Work out the finished part from the listing and answer in its coordinate system (mm). A direction names the side the tool comes from. Round coordinates to 2 decimals unless told otherwise and drop trailing zeros. Write each loop counter-clockwise with the first axis right and the second up, starting at its lowest first coordinate (ties: lowest second). Pieces come first, ordered by that corner, then holes.
1. Determine the mould class of faces 1 (the face through (9, -25, 0)), 2 (the face through (-4, -19, 2.85)), 3 (the face through (-2, -12, 3.5)) for opening direction Y: pulls with the +Y half, pulls with the -Y half, needs draft (parallel to the pull), parting line crosses it, or undercut.
2. Find section D-D (z = 0.5). Count the separate pieces of the cut face and the enclosed holes in it, and give its area (3 significant figures).
3. Straight lines are drawn through the part: probe 1 along Z at (x, y) = (-8.1, -19); probe 2 along Y at (x, z) = (-3, 3); probe 3 along Y at (x, z) = (-3.75, -1). For each, find the intervals that lie inside material, in ascending order.
4. Find section A-A (x = 0). Write down the section's boundary in (y, z), and give its area (3 significant figures).
5. Find section C-C (y = 0). Write down the section's boundary in (x, z), and give its area (3 significant figures).
6. A tool of negligible diameter and unlimited length cuts with its end or side. For faces 4 (the face through (2.53, -19.06, 0.33)), 5 (the face through (-1.49, -8.77, 0.94)), 6 (the face through (3.61, -25.02, -2.05)), 7 (the face through (7, -19, 0)), from which of +Z, -Z, +X, -X, +Y, -Y can it reach the whole face along a straight path? Write none if from no direction.
7. Find section B-B (y = -10). Write down the section's boundary in (x, z).
8. Flat-ended cylindrical pins translate along their axes: pin 1 Ø2 at (x, y) = (-5.5, 1) entering from +Z; pin 2 Ø6.5 at (y, z) = (-9, 0.5) entering from +X; pin 3 Ø2 at (y, z) = (-8.5, 1.5) entering from +X; pin 4 Ø10 at (x, y) = (0, 0) entering from +Z. Find the tip coordinate at first contact, or state that the pin passes through.
```python
from build123d import *

# Parameters (mm, degrees)
SKETCH1_R                      = 6.1
THICKNESS_DEPTH                = 3.5
BOTNUTCUT_START                = -2
SKETCH2_R                      = 2.85
BOTNUTCUT_DEPTH                = 2.6
SKETCH3_R                      = 1.55
BOTSCREWCUT_DEPTH              = 2
CUT_EXTRUDE1_START             = -7
CUT_EXTRUDE1_DEPTH             = 7
RAILNUTCUT_START               = -2
RAILNUTCUT_DEPTH               = 2.6
SKETCH7_R                      = 1.55
RAILSCREWCUT_DEPTH             = 2.6
RAILSCREWCUT_DIRECTION_2_REACH = 53.909
RAILNUTHEADCUT_REACH           = 56.409
RAILNUTHEADCUT_START           = -2.5
SKETCH8_R                      = 2.85
SKETCH9_W                      = 7
SKETCH9_H                      = 0.5
MOVEMENTCUT_DEPTH              = 7
SKETCH10_R                     = 4.5
BOSS_EXTRUDE1_DEPTH            = 3.5
CUT_EXTRUDE2_START             = -25
SKETCH11_W                     = 40
SKETCH11_H                     = 25
CUT_EXTRUDE2_DEPTH             = 25
SKETCH12_R                     = 8
BOSS_EXTRUDE2_DEPTH            = 10
CUT_EXTRUDE3_START             = -3
CUT_EXTRUDE3_DEPTH             = 4.1
SKETCH14_R                     = 2.55
CUT_EXTRUDE4_DEPTH             = 15
CUT_EXTRUDE5_REACH             = 34.79
SKETCH15_R                     = 1.55
CUT_EXTRUDE6_REACH             = 42.09
CUT_EXTRUDE6_START             = -7.3
SKETCH16_R                     = 2.85
CUT_EXTRUDE7_START             = -3
CUT_EXTRUDE7_DEPTH             = 2.6


with BuildPart() as part:
    # Sketch1 → Thickness (new, symmetric)
    with BuildSketch(Plane.XY):
        with BuildLine():
            Line((-13, -50), (13, -50))
            Line((13, -50), (8.424323952, -3.441041405))
            ThreePointArc((8.424323952, -3.441041405), (0, 9.1), (-8.424323952, -3.441041405))
            Line((-8.424323952, -3.441041405), (-13, -50))
        make_face()
        Circle(SKETCH1_R, mode=Mode.SUBTRACT)
    extrude(amount=THICKNESS_DEPTH, both=True)

    # Sketch2 → BotNutCut (cut)
    with BuildSketch(Plane.XZ.offset(50).offset(BOTNUTCUT_START)):
        with Locations((-7.5, 0)):
            Circle(SKETCH2_R)
        with BuildLine():
            Line((-10.790896534, 2.85), (-10.790896534, 0))
            Line((-10.790896534, 0), (-9.968172361, -1.42500007))
            ThreePointArc((-9.968172361, -1.42500007), (-9.96817242, 1.424999968), (-7.499999995, 2.85))
            Line((-7.499999995, 2.85), (-10.790896534, 2.85))
        make_face()
        with BuildLine():
            Line((-4.209103466, 2.85), (-7.499999995, 2.85))
            ThreePointArc((-7.499999995, 2.85), (-5.484745672, 2.015254324), (-4.65, 0))
            ThreePointArc((-4.65, 0), (-4.747111384, -0.737634237), (-5.031827556, -1.424999925))
            Line((-5.031827556, -1.424999925), (-4.209103466, 0))
            Line((-4.209103466, 0), (-4.209103466, 2.85))
        make_face()
        with BuildLine():
            ThreePointArc((-5.031827556, -1.424999925), (-6.074999963, -2.468172379), (-7.5, -2.85))
            Line((-7.5, -2.85), (-5.854551733, -2.85))
            Line((-5.854551733, -2.85), (-5.031827556, -1.424999925))
        make_face()
        with BuildLine():
            ThreePointArc((-7.5, -2.85), (-8.924999965, -2.468172421), (-9.968172361, -1.42500007))
            Line((-9.968172361, -1.42500007), (-9.145448267, -2.85))
            Line((-9.145448267, -2.85), (-7.5, -2.85))
        make_face()
        with BuildLine():
            ThreePointArc((7.5, -2.85), (6.074999995, -2.468172398), (5.031827593, -1.42499999))
            Line((5.031827593, -1.42499999), (5.854551733, -2.85))
            Line((5.854551733, -2.85), (7.5, -2.85))
        make_face()
        with BuildLine():
            ThreePointArc((9.968172375, -1.425000045), (8.924999978, -2.468172414), (7.5, -2.85))
            Line((7.5, -2.85), (9.145448267, -2.85))
            Line((9.145448267, -2.85), (9.968172375, -1.425000045))
        make_face()
        with BuildLine():
            Line((10.790896534, 2.85), (7.5, 2.85))
            ThreePointArc((7.5, 2.85), (9.515254326, 2.015254326), (10.35, 0))
            ThreePointArc((10.35, 0), (10.252888598, -0.737634304), (9.968172375, -1.425000045))
            Line((9.968172375, -1.425000045), (10.790896534, 0))
            Line((10.790896534, 0), (10.790896534, 2.85))
        make_face()
        with BuildLine():
            Line((4.209103466, 2.85), (4.209103466, 0))
            Line((4.209103466, 0), (5.031827593, -1.42499999))
            ThreePointArc((5.031827593, -1.42499999), (5.031827602, 1.425000005), (7.5, 2.85))
            Line((7.5, 2.85), (4.209103466, 2.85))
        make_face()
        with Locations((7.5, 0)):
            Circle(SKETCH2_R)
    extrude(amount=-BOTNUTCUT_DEPTH, mode=Mode.SUBTRACT)

    # Sketch3 → BotScrewCut (cut)
    with BuildSketch(Plane.XZ.offset(50)):
        with Locations(Location((-7.5, 0, 0), (0, 0, 270))):
            Circle(SKETCH3_R)
        with Locations(Location((7.5, 0, 0), (0, 0, 270))):
            Circle(SKETCH3_R)
    extrude(amount=-BOTSCREWCUT_DEPTH, mode=Mode.SUBTRACT)

    # Sketch5 → Cut-Extrude1 (cut)
    with BuildSketch(Plane.XY.offset(3.5).offset(CUT_EXTRUDE1_START)):
        with BuildLine():
            ThreePointArc((0.5, -6.079473661), (0, -6.1), (-0.5, -6.079473661))
            Line((-0.5, -6.079473661), (-0.5, -12.924568984))
            ThreePointArc((-0.5, -12.924568984), (0, -23.1), (0.5, -12.924568984))
            Line((0.5, -12.924568984), (0.5, -6.079473661))
        make_face()
    extrude(amount=CUT_EXTRUDE1_DEPTH, mode=Mode.SUBTRACT)

    # Sketch6 → RailNutCut (cut)
    with BuildSketch(Plane(origin=(-0.5, 0, 0), x_dir=(0, 0, -1), z_dir=(1, 0, 0)).offset(RAILNUTCUT_START)):
        Polygon((0, -13.290896534), (2.85, -11.645448267), (2.85, -8.354551733), (0, -6.709103466), (-2.85, -6.709103466), (-2.85, -13.290896534), align=None)
    extrude(amount=-RAILNUTCUT_DEPTH, mode=Mode.SUBTRACT)

    # Sketch7 → RailScrewCut (cut)
    with BuildSketch(Plane(origin=(-0.5, 0, 0), x_dir=(0, 0, -1), z_dir=(1, 0, 0))):
        with Locations(Location((0, -10, 0), (0, 0, 270))):
            Circle(SKETCH7_R)
    extrude(amount=-RAILSCREWCUT_DEPTH, mode=Mode.SUBTRACT)

    # RailScrewCut direction 2: up to this plane
    railscrewcut_direction_2_end = Plane(origin=(13, -50, 3.5), z_dir=(-0.9952055153223801, -0.09780583966162733, 0))
    # Sketch7 → RailScrewCut direction 2 (cut, up to the surface)
    with BuildSketch(Plane(origin=(-0.5, 0, 0), x_dir=(0, 0, -1), z_dir=(1, 0, 0)), mode=Mode.PRIVATE) as railscrewcut_direction_2_sk1:
        with Locations(Location((0, -10, 0), (0, 0, 270))):
            Circle(SKETCH7_R)
    railscrewcut_direction_2_tool1 = split(extrude(railscrewcut_direction_2_sk1.sketch, amount=RAILSCREWCUT_DIRECTION_2_REACH, mode=Mode.PRIVATE), bisect_by=railscrewcut_direction_2_end, keep=Keep.BOTH, mode=Mode.PRIVATE)
    add(railscrewcut_direction_2_tool1.solids().sort_by_distance((-0.5, -10, 0))[0], mode=Mode.SUBTRACT)

    # RailNutHeadCut: up to this plane
    railnutheadcut_end = Plane(origin=(13, -50, 3.5), z_dir=(-0.9952055153223801, -0.09780583966162733, 0))
    # Sketch8 → RailNutHeadCut (cut, up to the surface)
    with BuildSketch(Plane.ZY.offset(-0.5).offset(RAILNUTHEADCUT_START), mode=Mode.PRIVATE) as railnutheadcut_sk1:
        with Locations(Location((0, -10, 0), (0, 0, 270))):
            Circle(SKETCH8_R)
    railnutheadcut_tool1 = split(extrude(railnutheadcut_sk1.sketch, amount=-RAILNUTHEADCUT_REACH, mode=Mode.PRIVATE), bisect_by=railnutheadcut_end, keep=Keep.BOTH, mode=Mode.PRIVATE)
    add(railnutheadcut_tool1.solids().sort_by_distance((3, -10, 0))[0], mode=Mode.SUBTRACT)

    # Sketch9 → MovementCut (cut)
    with BuildSketch(Plane.XY.offset(3.5)):
        with Locations((7.5, -18.75)):
            Rectangle(SKETCH9_W, SKETCH9_H)
    extrude(amount=-MOVEMENTCUT_DEPTH, mode=Mode.SUBTRACT)

    # Sketch10 → Boss-Extrude1 (add, symmetric)
    with BuildSketch(Plane.XY):
        with BuildLine():
            Line((-0.5, -13.527864045), (-0.5, -12.924568984))
            ThreePointArc((-0.5, -12.924568984), (-3.780537731, -21.42308844), (5.0009999, -19))
            Line((5.0009999, -19), (4.387482194, -19))
            ThreePointArc((4.387482194, -19), (-3.356217727, -20.997632828), (-0.5, -13.527864045))
        make_face()
        with Locations((0, -18)):
            Circle(SKETCH10_R)
    extrude(amount=BOSS_EXTRUDE1_DEPTH, both=True)

    # Sketch11 → Cut-Extrude2 (cut)
    with BuildSketch(Plane(origin=(0, 0, 0), x_dir=(1, 0, 0), z_dir=(0, 1, 0)).offset(CUT_EXTRUDE2_START)):
        Rectangle(SKETCH11_W, SKETCH11_H)
    extrude(amount=-CUT_EXTRUDE2_DEPTH, mode=Mode.SUBTRACT)

    # Sketch12 → Boss-Extrude2 (add)
    with BuildSketch(Plane(origin=(0, -20, 0), x_dir=(1, 0, 0), z_dir=(0, 1, 0))):
        with Locations(Location((0, 0, 0), (0, 0, 270))):
            Circle(SKETCH12_R)
    extrude(amount=-BOSS_EXTRUDE2_DEPTH)

    # Sketch13 → Cut-Extrude3 (cut)
    with BuildSketch(Plane(origin=(0, -20, 0), x_dir=(1, 0, 0), z_dir=(0, 1, 0)).offset(CUT_EXTRUDE3_START)):
        Polygon((-4.792007234, 0), (-4.792007234, -4.15), (4.792007234, -4.15), (4.792007234, 0), (2.396003617, 4.15), (-2.396003617, 4.15), align=None)
    extrude(amount=-CUT_EXTRUDE3_DEPTH, mode=Mode.SUBTRACT)

    # Sketch14 → Cut-Extrude4 (cut)
    with BuildSketch(Plane.XZ.offset(30)):
        with Locations(Location((0, 0, 0), (0, 0, 270))):
            Circle(SKETCH14_R)
    extrude(amount=-CUT_EXTRUDE4_DEPTH, mode=Mode.SUBTRACT)

    # Cut-Extrude5: up to this plane
    cut_extrude5_end = Plane(origin=(-13, -50, 3.5), z_dir=(0.9952055153223801, -0.09780583966162733, 0))
    # Sketch15 → Cut-Extrude5 (cut, up to the surface)
    with BuildSketch(Plane(origin=(0, 0, 0), x_dir=(0, 0, -1), z_dir=(1, 0, 0)), mode=Mode.PRIVATE) as cut_extrude5_sk1:
        with Locations((0, -19)):
            Circle(SKETCH15_R)
    cut_extrude5_tool1 = split(extrude(cut_extrude5_sk1.sketch, amount=-CUT_EXTRUDE5_REACH, mode=Mode.PRIVATE), bisect_by=cut_extrude5_end, keep=Keep.BOTH, mode=Mode.PRIVATE)
    add(cut_extrude5_tool1.solids().sort_by_distance((0, -19, 0))[0], mode=Mode.SUBTRACT)

    # Cut-Extrude6: up to this plane
    cut_extrude6_end = Plane(origin=(-13, -50, 3.5), z_dir=(0.9952055153223801, -0.09780583966162733, 0))
    # Sketch16 → Cut-Extrude6 (cut, up to the surface)
    with BuildSketch(Plane(origin=(0, 0, 0), x_dir=(0, 0, -1), z_dir=(1, 0, 0)).offset(CUT_EXTRUDE6_START), mode=Mode.PRIVATE) as cut_extrude6_sk1:
        with Locations((0, -19)):
            Circle(SKETCH16_R)
    cut_extrude6_tool1 = split(extrude(cut_extrude6_sk1.sketch, amount=-CUT_EXTRUDE6_REACH, mode=Mode.PRIVATE), bisect_by=cut_extrude6_end, keep=Keep.BOTH, mode=Mode.PRIVATE)
    add(cut_extrude6_tool1.solids().sort_by_distance((-7.3, -19, 0))[0], mode=Mode.SUBTRACT)

    # Sketch17 → Cut-Extrude7 (cut)
    with BuildSketch(Plane(origin=(0, 0, 0), x_dir=(0, 0, -1), z_dir=(1, 0, 0)).offset(CUT_EXTRUDE7_START)):
        Polygon((-2.85, -15.709103466), (-2.85, -22.290896534), (0, -22.290896534), (2.85, -20.645448267), (2.85, -17.354551733), (0, -15.709103466), align=None)
    extrude(amount=-CUT_EXTRUDE7_DEPTH, mode=Mode.SUBTRACT)


solid = part.part
```
Worked answers:
1. face 1: pulls with the -Y half
1. face 2: undercut
1. face 3: needs draft
2. separate pieces: 3
2. enclosed holes: 0
2. area: 352 mm2
3. probe 1: z = -3.5 to -2.85, 2.85 to 3.5
3. probe 2: y = -30 to -27.1, -23 to -5.31, 5.31 to 8.59
3. probe 3: y = -30 to -27.1, -23 to -21.71, -16.29 to -12.71, -7.29 to -4.81, 4.81 to 8.29
4. outline: (-30, -8) - (-20, -8) - (-20, -3.5) - (-13.5, -3.5) - (-13.5, 3.5) - (-20, 3.5) - (-20, 8) - (-30, 8) - (-30, 2.55) - (-27.1, 2.55) - (-27.1, 4.15) - (-23, 4.15) - (-23, 2.55) - (-15, 2.55) - (-15, -2.55) - (-23, -2.55) - (-23, -4.15) - (-27.1, -4.15) - (-27.1, -2.55) - (-30, -2.55) - close; (6.1, -3.5) - (9.1, -3.5) - (9.1, 3.5) - (6.1, 3.5) - close
4. area: 137 mm2
5. outline: (-9.1, -3.5) - (-6.1, -3.5) - (-6.1, 3.5) - (-9.1, 3.5) - close; (6.1, -3.5) - (9.1, -3.5) - (9.1, 3.5) - (6.1, 3.5) - close
5. area: 42.0 mm2
6. face 4: -Y
6. face 5: +X
6. face 6: none
6. face 7: +Z, -Z, +X
7. outline: (-9.07, -3.5) - (-0.5, -3.5) - (-0.5, -1.55) - (-2.5, -1.55) - (-2.5, -2.85) - (-5.1, -2.85) - (-5.1, 2.85) - (-2.5, 2.85) - (-2.5, 1.55) - (-0.5, 1.55) - (-0.5, 3.5) - (-9.07, 3.5) - close; (0.5, -3.5) - (9.07, -3.5) - (9.07, -2.85) - (3, -2.85) - (3, -1.55) - (0.5, -1.55) - close; (0.5, 1.55) - (3, 1.55) - (3, 2.85) - (9.07, 2.85) - (9.07, 3.5) - (0.5, 3.5) - close
8. pin 1: stops at z = 3.5
8. pin 2: stops at x = 9.24
8. pin 3: stops at x = 8.93
8. pin 4: passes through
